For this review, take the finished solid that the model builds, in its own axes (mm). A direction names the side the tool comes from. Round coordinates to 2 decimals unless told otherwise and drop trailing zeros. Write each loop counter-clockwise with the first axis right and the second up, starting at its lowest first coordinate (ties: lowest second). Pieces come first, ordered by that corner, then holes. Notation, with made-up numbers: (73, -8.75) -> (79, -8.75) arc R24 ccw to (79, 15.25) -> close; hole circle Ø3 at (-32.5, 30.25). An arc over 180 degrees is marked (long way). Answer in a Markdown table with one row per item.
from build123d import *

# Parameters (mm, degrees)
F2_DEPTH = 400
F5_DEPTH = 10
F8_R     = 2


with BuildPart() as f2:
    # F1 (on Front) → F2 (new body)
    with BuildSketch(Plane.XZ):
        Polygon((-199.8697698991, -1.5957240637), (-199.8697698991, -9.5957240637), (-174.8697698991, -9.5957240637), (-110, 120.4042759363), (-110, 290.4042759363), (0, 290.4042759363), (0, 298.4042759363), (-118, 298.4042759363), (-118, 122.289434411), (-179.8184748013, -1.5957240637), align=None)
        Polygon((0, 298.4042759363), (0, 290.4042759363), (110, 290.4042759363), (110, 120.4042759363), (174.8697698991, -9.5957240637), (199.8697698991, -9.5957240637), (199.8697698991, -1.5957240637), (179.8184748013, -1.5957240637), (118, 122.289434411), (118, 298.4042759363), align=None)
    extrude(amount=F2_DEPTH)


with BuildPart() as f5:
    # F4 (on offset) → F5 (new body)
    with BuildSketch(Plane.XZ.offset(400)):
        Polygon((118, 298.4042759363), (-118, 298.4042759363), (-118, 122.289434411), (-179.548561573, -1.5957240637), (-199.8697698991, -1.5957240637), (-199.8697698991, -9.5957240637), (199.8697698991, -9.5957240637), (199.8697698991, -1.5957240637), (179.7748506069, -1.5957240637), (118, 122.289434411), align=None)
    extrude(amount=-F5_DEPTH)

    # F6: cut F2
    add(f2.part, mode=Mode.SUBTRACT)

    # F7: union F2
    add(f2.part)

    # F8
    f8_edges = [f5.edges().sort_by_distance(p)[0] for p in [
        (-189.844122, -400, -1.595724),
        (-199.86977, -400, -5.595724),
        (0, -400, -9.595724),
        (199.86977, -400, -5.595724),
        (189.844122, -400, -1.595724),
        (148.909237, -400, 60.346855),
        (118, -400, 210.346855),
        (0, -400, 298.404276),
        (-118, -400, 210.346855),
        (-148.909237, -400, 60.346855),
    ]]
    fillet(f8_edges, radius=F8_R)


solid = f5.part
1) For faces 4 (the flat face through (-2, -390, 109)), 5 (the flat face through (190, -196, -1.596)), 6 (the flat face through (2, -196, 298.404)), 7 (the flat face through (-190, -196, -1.596)), list the 3-axis set-ups (+Z, -Z, +X, -X, +Y, -Y) from which the entire face can be reached by the end or side of a thin tool; tool diameter is ignored.
Solved:
| item | result |
|---|---|
| face 4 | -Z, +Y |
| face 5 | +Z, +X, +Y, -Y |
| face 6 | +Z, +X, -X, +Y, -Y |
| face 7 | +Z, -X, +Y, -Y |
2) For line 1 (X direction, y = -261, z = 152); line 2 (Z direction, x = -59, y = -201); line 3 (X direction, y = -98, z = 65), list the stretches that pass through material, from the lowest coordinate up. Write a range as [from, to].
Solved:
| item | result |
|---|---|
| line 1 | [-118, -110], [110, 118] |
| line 2 | [290.4, 298.4] |
| line 3 | [-146.59, -137.65], [137.65, 146.59] |
3) Mouldability with a two-part tool opening along X and no side actions: class faces 1 (the flat face through (110, -192, 207)), 2 (the cylindrical face through (148.104, -399.43, 60.614)), 3 (the flat face through (-179, -198, -9.596)) as pulls with the +X half, pulls with the -X half, needs draft (parallel to the pull), parting line crosses it, or undercut.
Solved:
| item | result |
|---|---|
| face 1 | undercut |
| face 2 | pulls with the +X half |
| face 3 | needs draft |
4) Consider section C-C on x = -90.5. State the section outline as (y, z) points, then the cut area to 3 significant figures.
Solved:
| item | result |
|---|---|
| outline | (-400, -7.6) arc R2 ccw to (-398, -9.6) -> (-390, -9.6) -> (-390, 290.4) -> (0, 290.4) -> (0, 298.4) -> (-398, 298.4) arc R2 ccw to (-400, 296.4) -> close |
| area | 6,200 mm² |
5) Consider section B-B on z = 248. State the section outline as (x, y) points, then the cut area to 3 significant figures.
Solved:
| item | result |
|---|---|
| outline | (-118, -398) arc R2 ccw to (-116, -400) -> (116, -400) arc R2 ccw to (118, -398) -> (118, 0) -> (110, 0) -> (110, -390) -> (-110, -390) -> (-110, 0) -> (-118, 0) -> close |
| area | 8,600 mm² |
6) Clearance check with flat-ended pins moving along their axes: pin 1 Ø2 at (x, y) = (-134, -267) entering from -Z; pin 2 Ø8 at (x, z) = (80.5, 89.5) entering from +Y; pin 3 Ø4 at (y, z) = (-175.5, 222) entering from -X. State where each tip first meets the part, or that it passes through.
Solved:
| item | result |
|---|---|
| pin 1 | z = 70.3 |
| pin 2 | y = -390 |
| pin 3 | x = -118 |
7) Consider section A-A on y = -92. State the section outline as (x, z) points, then the cut area to 3 significant figures.
Solved:
| item | result |
|---|---|
| outline | (-199.87, -9.6) -> (-174.87, -9.6) -> (-110, 120.4) -> (-110, 290.4) -> (110, 290.4) -> (110, 120.4) -> (174.87, -9.6) -> (199.87, -9.6) -> (199.87, -1.6) -> (179.82, -1.6) -> (118, 122.29) -> (118, 298.4) -> (-118, 298.4) -> (-118, 122.29) -> (-179.82, -1.6) -> (-199.87, -1.6) -> close |
| area | 7,220 mm² |
